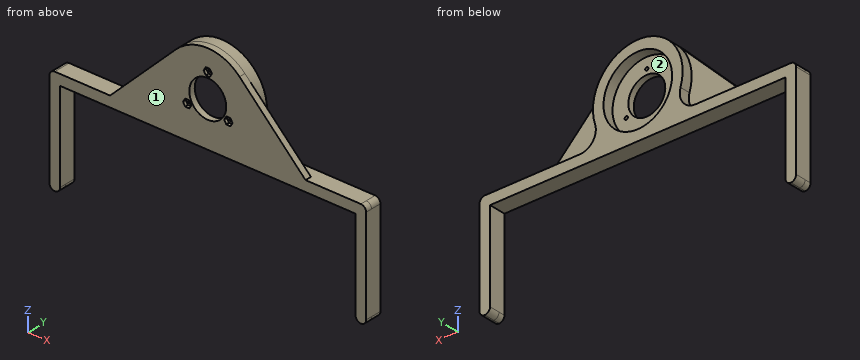
from build123d import *

# Parameters (mm, degrees)
SKETCH1_R           = 32.5
BOSS_EXTRUDE1_DEPTH = 10
FILLET1_R           = 5
FILLET2_R           = 15
BOSS_EXTRUDE2_START = 6
SKETCH2_R           = 1.55
SKETCH2_R_2         = 17.5
BOSS_EXTRUDE2_DEPTH = 6
CUT_EXTRUDE1_DEPTH  = 3


with BuildPart() as part:
    # Sketch1 → Boss-Extrude1 (new body)
    with BuildSketch(Plane(origin=(0, 0, 0), x_dir=(1, 0, 0), z_dir=(0, 1, 0))):
        with BuildLine():
            Line((0, 42.5), (140, 42.5))
            Line((140, 42.5), (140, 132.5))
            Line((140, 132.5), (150, 132.5))
            Line((150, 132.5), (150, 42.5))
            Line((150, 42.5), (150, 32.5))
            Line((150, 32.5), (27.386127875, 32.5))
            ThreePointArc((27.386127875, 32.5), (0, -42.5), (-27.386127875, 32.5))
            Line((-27.386127875, 32.5), (-150, 32.5))
            Line((-150, 32.5), (-150, 42.5))
            Line((-150, 42.5), (-150, 132.5))
            Line((-150, 132.5), (-140, 132.5))
            Line((-140, 132.5), (-140, 42.5))
            Line((-140, 42.5), (0, 42.5))
        make_face()
        with Locations(Location((0, 0, 0), (0, 0, 270))):
            Circle(SKETCH1_R, mode=Mode.SUBTRACT)
    extrude(amount=BOSS_EXTRUDE1_DEPTH)

    # Fillet1
    fillet1_edges = [part.edges().sort_by_distance(p)[0] for p in [
        (150, 5, -132.5),
        (140, 5, -132.5),
        (150, 5, -32.5),
        (-150, 5, -32.5),
        (-140, 5, -132.5),
        (-150, 5, -132.5),
    ]]
    fillet(fillet1_edges, radius=FILLET1_R - 0.0001)  # a hair under: the kernel refuses the full size

    # Fillet2
    fillet2_edges = [part.edges().sort_by_distance(p)[0] for p in [
        (27.386127875, 5, -32.5),
        (-27.386127875, 5, -32.5),
    ]]
    fillet(fillet2_edges, radius=FILLET2_R)

    # Sketch2 → Boss-Extrude2 (add)
    with BuildSketch(Plane.XZ.offset(BOSS_EXTRUDE2_START)):
        with BuildLine():
            Line((-30.0520382, 30.0520382), (-92.604076401, -32.5))
            Line((-92.604076401, -32.5), (-145, -32.5))
            ThreePointArc((-145, -32.5), (-148.535533906, -33.964466094), (-150, -37.5))
            Line((-150, -37.5), (-150, -127.5))
            ThreePointArc((-150, -127.5), (-148.535533906, -131.035533906), (-145, -132.5))
            ThreePointArc((-145, -132.5), (-141.464466094, -131.035533906), (-140, -127.5))
            Line((-140, -127.5), (-140, -42.5))
            Line((-140, -42.5), (140, -42.5))
            Line((140, -42.5), (140, -127.5))
            ThreePointArc((140, -127.5), (141.464466094, -131.035533906), (145, -132.5))
            ThreePointArc((145, -132.5), (148.535533906, -131.035533906), (150, -127.5))
            Line((150, -127.5), (150, -37.5))
            ThreePointArc((150, -37.5), (148.535533906, -33.964466094), (145, -32.5))
            Line((145, -32.5), (92.604076401, -32.5))
            Line((92.604076401, -32.5), (30.0520382, 30.0520382))
            ThreePointArc((30.0520382, 30.0520382), (0, 42.5), (-30.0520382, 30.0520382))
        make_face()
        with Locations(Location((0, 22.5, 0), (0, 0, 270))):
            Circle(SKETCH2_R, mode=Mode.SUBTRACT)
        with Locations(Location((19.485571585, -11.25, 0), (0, 0, 270))):
            Circle(SKETCH2_R, mode=Mode.SUBTRACT)
        with Locations(Location((-19.485571585, -11.25, 0), (0, 0, 270))):
            Circle(SKETCH2_R, mode=Mode.SUBTRACT)
        with Locations(Location((0, 0, 0), (0, 0, 270))):
            Circle(SKETCH2_R_2, mode=Mode.SUBTRACT)
    extrude(amount=-BOSS_EXTRUDE2_DEPTH)

    # Sketch4 → Cut-Extrude1 (cut)
    with BuildSketch(Plane.XZ.offset(6)):
        Polygon((17.519605061, -14.655153906), (21.451538109, -14.655153906), (23.417504634, -11.25), (21.451538109, -7.844846094), (17.519605061, -7.844846094), (15.553638537, -11.25), align=None)
        Polygon((3.931933048, 22.5), (1.965966524, 25.905153906), (-1.965966524, 25.905153906), (-3.931933048, 22.5), (-1.965966524, 19.094846094), (1.965966524, 19.094846094), align=None)
        Polygon((-21.451538109, -7.844846094), (-23.417504634, -11.25), (-21.451538109, -14.655153906), (-17.519605061, -14.655153906), (-15.553638537, -11.25), (-17.519605061, -7.844846094), align=None)
    extrude(amount=-CUT_EXTRUDE1_DEPTH, mode=Mode.SUBTRACT)


solid = part.part
Input: part model. Units: mm. Frame: model coordinates. Face numbers are marked on the shaded views. Coordinates: 2 decimals unless noted, no trailing zeros. Order: outer loops, then holes, each group sorted by start corner. A loop starts at its lowest first (then second) coordinate and runs counter-clockwise, first axis right, second up. Notation, with made-up numbers: M 75,25.5 L 96,25.5 A32 cw 96,60.5 Z; hole C 14,-26.5 d4. An arc over 180 degrees is marked long. One line per question, with ' | ' between items.
Item 1: Draft query along Z for the marked faces 1 and 2. Return one class per face: released by +Z, released by -Z, zero draft, split by the parting line, or undercut.
Geometry results:
face 1: zero draft | face 2: undercut
Item 2: Section C-C (z = 13). Output: boundary loops of the cut face in (x, y), then the cut area to 3 significant figures.
Geometry results:
outline: M -47.1,-6 L -11.72,-6 L -11.72,0 L -29.79,0 L -29.79,10 L -40.46,10 L -40.46,0 L -47.1,0 Z; M 11.72,-6 L 47.1,-6 L 47.1,0 L 40.46,0 L 40.46,10 L 29.79,10 L 29.79,0 L 11.72,0 Z | area: 638 mm^2
Item 3: Section D-D (x = 77). Output: boundary loops of the cut face in (y, z), then the cut area to 3 significant figures.
Geometry results:
outline: M -6,-42.5 L 10,-42.5 L 10,-32.5 L 0,-32.5 L 0,-16.9 L -6,-16.9 Z | area: 254 mm^2
Item 4: Section A-A (z = -116). Output: boundary loops of the cut face in (x, y), then the cut area to 3 significant figures.
Geometry results:
outline: M -150,-6 L -140,-6 L -140,10 L -150,10 Z; M 140,-6 L 150,-6 L 150,10 L 140,10 Z | area: 320 mm^2
Item 5: Ray query, line 1 along X through (y, z) = (-1, -11.25); line 2 along X through (y, z) = (3.75, -104); line 3 along Y through (x, z) = (54.5, -27.5). Return the intervals inside material, ascending.
Geometry results:
line 1: x = -71.35 to -21.04, -17.94 to -13.4, 13.4 to 17.94, 21.04 to 71.35 | line 2: x = -150 to -140, 140 to 150 | line 3: y = -6 to 0
Item 6: Pin query (flat end, axial travel): pin 1 (3.5 mm diameter, centred on x = -19.49, z = -11.25, fed in from +Y); pin 2 (3.5 mm diameter, centred on x = -19, z = -11.5, fed in from -Y); pin 3 (2 mm diameter, centred on x = 83.5, y = 0.5, fed in from +Z). Return the tip coordinate at first contact, or that it passes through.
Geometry results:
pin 1: stops at y = 0 | pin 2: stops at y = -3 | pin 3: stops at z = -22.53
